Can you work these out from the model? Positions are in its coordinate system, mm. Face numbers are marked on the shaded views. Coordinates: 2 decimals unless noted, no trailing zeros. Loops run counter-clockwise (first coordinate to the right, second up) from the corner with the lowest first, then second, coordinate; pieces in that order, holes last. Notation, with made-up numbers: (19, -17) -> (71, -17) arc R25 ccw to (71, 8) -> close; hole circle Ø11 at (-4, 51.5). An arc over 180 degrees is marked (long way). Use one line per item in the form item = value. Start each with the question number.
(1) Imagine slicing it at C-C (z = -10.5). List the corners of the cut face in (x, y) for me, plus the area to 3 significant figures.
(2) Imagine slicing it at A-A (y = -4). List the corners of the cut face in (x, z) for me, plus the area to 3 significant figures.
(3) I'm going to push a flat-ended pin straight in: pin 1 (1 mm diameter, centred on x = 68.5, y = -5.5, fed in from +Z). Where does the tip first touch, or does it pass through?
(4) Thinking about a two-plate mould opening in Z: for the marked faces 1 and 2, which applies, released by +Z, released by -Z, zero draft, split by the parting line, or undercut?
(5) Imagine slicing it at B-B (x = 445). List the corners of the cut face in (y, z) for me (1 decimal), plus the area to 3 significant figures.
(6) I need wall thicknesses on line 1 (Y direction, x = 302.5, z = -7.5); line 2 (Z direction, x = 210.5, y = -2.25); line 3 (Z direction, x = 62, y = -7.5). Which ranges of each line are inside material? Lowest first, please. Write a range as [from, to].
Autodesk Inventor part; units mm, degrees
ref_plane "YZ Plane" through (0, 0, 0) normal (1, 0, 0) x (0, 1, 0)
ref_plane "XZ Plane" through (0, 0, 0) normal (0, 1, 0) x (-1, 0, 0)
ref_plane "XY Plane" through (0, 0, 0) normal (0, 0, 1) x (1, 0, 0)
sketch "Sketch1" plane through (0, 0, 0) normal (1, 0, 0) x (0, 1, 0)
  line L0 (0, -0.4446) -> (0, -37.6554)
  line L1 (-0.4178, 0.1521) -> (-6.7426, 2.4541)
  line L2 (-7.4463, 2.2656) -> (-9.6095, -0.3124)
  line L3 (-0.4178, -38.2521) -> (-6.7426, -40.5541)
  line L4 (-7.4463, -40.3656) -> (-9.6095, -37.7876)
  line L5 (-8.0529, -36.4814) -> (-6.8042, -37.9695)
  line L6 (-6.1006, -38.158) -> (-2.4498, -36.8293)
  line L7 (-2.032, -36.2325) -> (-2.032, -1.8675)
  line L8 (-2.4498, -1.2707) -> (-6.1006, 0.058)
  line L9 (-6.8042, -0.1305) -> (-8.0529, -1.6186)
  line L10 (-9.6095, -0.3124) -> (-8.0529, -1.6186)
  line L11 (-8.0529, -36.4814) -> (-9.6095, -37.7876)
  arc A0 (0, -0.4446) -> (-0.4178, 0.1521) centre (-0.635, -0.4446) ccw
  arc A1 (-2.032, -1.8675) -> (-2.4498, -1.2707) centre (-2.667, -1.8675) ccw
  arc A2 (-6.1006, 0.058) -> (-6.8042, -0.1305) centre (-6.3178, -0.5387) ccw
  arc A3 (-6.7426, 2.4541) -> (-7.4463, 2.2656) centre (-6.9598, 1.8574) ccw
  arc A4 (-0.4178, -38.2521) -> (0, -37.6554) centre (-0.635, -37.6554) ccw
  arc A5 (-2.4498, -36.8293) -> (-2.032, -36.2325) centre (-2.667, -36.2325) ccw
  arc A6 (-6.8042, -37.9695) -> (-6.1006, -38.158) centre (-6.3178, -37.5613) ccw
  arc A7 (-7.4463, -40.3656) -> (-6.7426, -40.5541) centre (-6.9598, -39.9574) ccw
  point P0 (0, 0)
  point P1 (0, -38.1)
  point P2 (-7.1605, 2.6062)
  point P3 (-7.1605, -40.7062)
  point P4 (-6.5184, -38.3101)
  point P5 (-6.5184, 0.2101)
  dimension "d7" = 7.62
  dimension "d8" = 3.81
  dimension "d9" = 110
  dimension "d10" = 110
  dimension "d11" = 7.62
  dimension "d12" = 3.81
  dimension "d13" = 110
  dimension "d14" = 110
  dimension "d15" = 38.1
  dimension "d16" = 2.032
  dimension "d17" = 2.3872
  dimension "d18" = 2.3872
  dimension "d19" = 0.635
extrude "Extrusion1" add sketch "Sketch1" along normal blind 609.6
properties part number "the inside for the 2nd slider part"
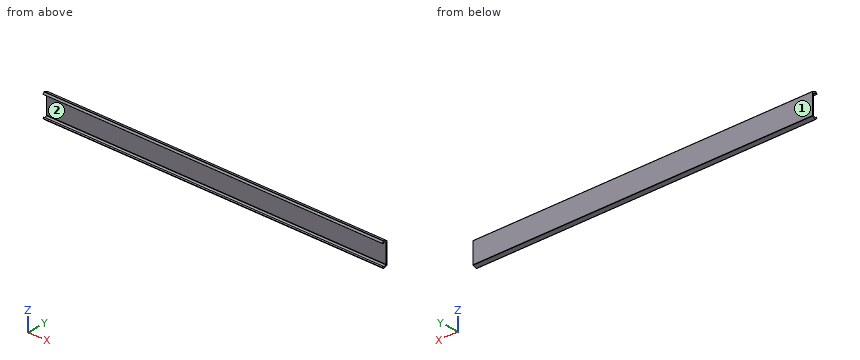
Worked out:
q1.outline = (0, -2.03) -> (609.6, -2.03) -> (609.6, 0) -> (0, 0) -> close
q1.area = 1,240 mm2
q2.outline = (0, -39.56) -> (609.6, -39.56) -> (609.6, -37.39) -> (0, -37.39) -> close; (0, -0.71) -> (609.6, -0.71) -> (609.6, 1.46) -> (0, 1.46) -> close
q2.area = 2,640 mm2
q3.pin_1 = 2.18
q4.face_1 = zero draft
q4.face_2 = undercut
q5.outline = (-9.6, -37.8) -> (-7.4, -40.4) arc R0.6 ccw to (-6.7, -40.6) -> (-0.4, -38.3) arc R0.6 ccw to (0, -37.7) -> (0, -0.4) arc R0.6 ccw to (-0.4, 0.2) -> (-6.7, 2.5) arc R0.6 ccw to (-7.4, 2.3) -> (-9.6, -0.3) -> (-8.1, -1.6) -> (-6.8, -0.1) arc R0.6 cw to (-6.1, 0.1) -> (-2.4, -1.3) arc R0.6 cw to (-2, -1.9) -> (-2, -36.2) arc R0.6 cw to (-2.4, -36.8) -> (-6.1, -38.2) arc R0.6 cw to (-6.8, -38) -> (-8.1, -36.5) -> close
q5.area = 112 mm2
q6.line_1 = [-2.03, 0]
q6.line_2 = [-38.92, -36.71], [-1.39, 0.82]
q6.line_3 = [-40.3, -37.14], [-0.96, 2.2]
